Design review of the part shown in the three views and the two pictorial views. Dimensions are in mm from the part's minimum x, y and z. A direction names the side the tool comes from. Coordinates: 2 decimals unless noted, no trailing zeros. Write each loop counter-clockwise with the first axis right and the second up, starting at its lowest first coordinate (ties: lowest second). Pieces come first, ordered by that corner, then holes. Notation, with made-up numbers: (36, 21.25) -> (45, 21.25) arc R25 ccw to (45, 36.25) -> close; hole circle Ø5 at (-15.5, 10.25). An arc over 180 degrees is marked (long way). Write each question's results on one line, items separated by ' | '.
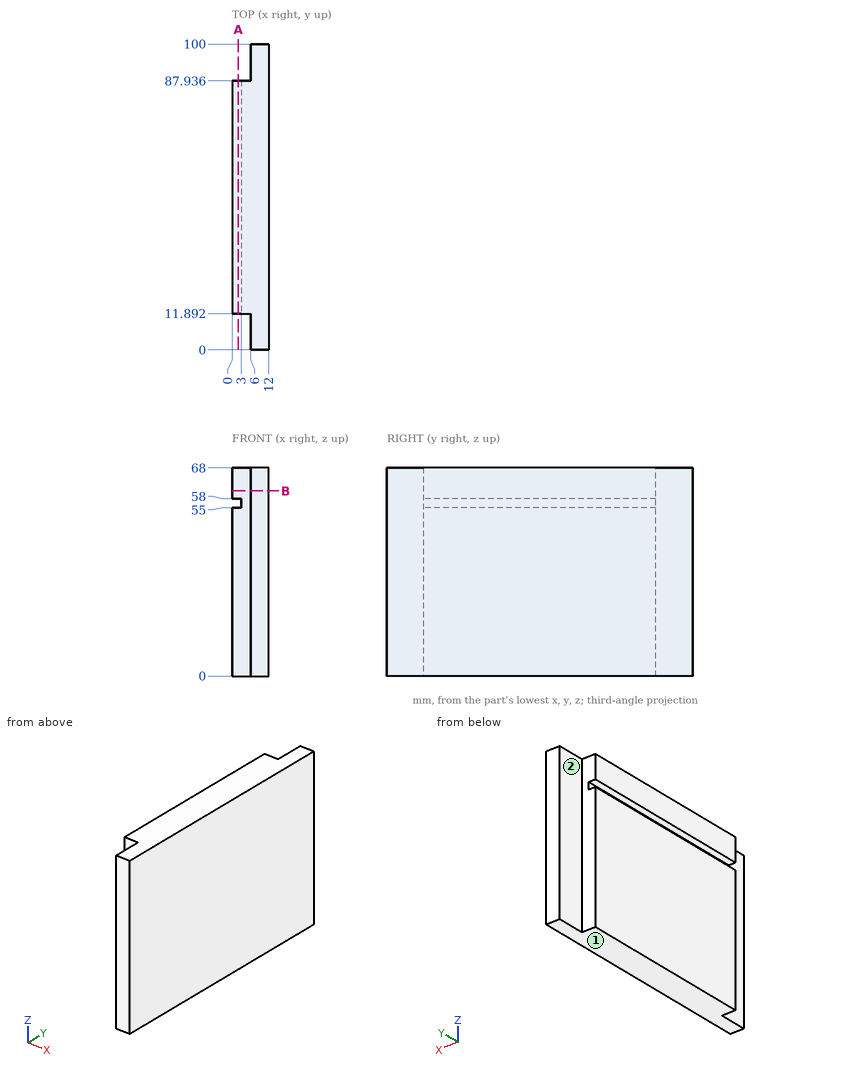
Q1. Add section A-A (x = 2). Write out the cut boundary in (y, z) (1 decimal).
Solution:
outline: (11.9, 0) -> (87.9, 0) -> (87.9, 55) -> (11.9, 55) -> close; (11.9, 58) -> (87.9, 58) -> (87.9, 68) -> (11.9, 68) -> close
Q2. Clearance check with flat-ended pins moving along their axes: P1, Ø5, axis at x = 2.5, z = 47.5, coming from the +Y side (1 decimal); P2, Ø1.8, axis at x = 2, z = 36.5, coming from the -Y side; P3, Ø6, axis at y = 93, z = 24, coming from the -X side. State where each tip first meets the part, or that it passes through.
Solution:
P1: y = 87.9 | P2: y = 11.89 | P3: x = 6
Q3. Machinability: for the marked faces 1 and 2, which of the approach directions +Z, -Z, +X, -X, +Y, -Y give a long, thin tool a straight path to every point of the face, cutting with its end or side? Answer none if there is none.
Solution:
face 1: -Z, +X, -X, +Y, -Y | face 2: +Z, -Z, -X, +Y
Q4. Add section B-B (z = 60.5). Write out the cut boundary in (x, y) (1 decimal), plus the area to 3 significant figures.
Solution:
outline: (0, 11.9) -> (6, 11.9) -> (6, 0) -> (12, 0) -> (12, 100) -> (6, 100) -> (6, 87.9) -> (0, 87.9) -> close | area: 1,060 mm²
Q5. For line 1 (Z direction, x = 1.5, y = 82); line 2 (X direction, y = 88.5, z = 15); line 3 (Y direction, x = 2, z = 29.5) (1 decimal), list the stretches that pass through material, from the lowest coordinate up. Write a range as from..to.
Solution:
line 1: 0..55, 58..68 | line 2: 6..12 | line 3: 11.9..87.9
